Part model, mm, in its own coordinate system. A direction names the side the tool comes from. Give positions to 0.01 mm unless a question says otherwise; leave off trailing zeros. Write each loop counter-clockwise with the first axis right and the second up, starting at its lowest first coordinate (ties: lowest second). Pieces come first, ordered by that corner, then holes.
```python
from build123d import *

# Parameters (mm, degrees)
F0_R     = 1.778
F1_DEPTH = 2.159
F2_DEPTH = 6.35


with BuildPart() as f1:
    # F0 (on Front) → F1 (new body)
    with BuildSketch(Plane.XZ):
        Polygon((-13.906726, -6.464459), (-13.906726, -13.791269), (7.429274, -13.791269), (7.429274, -6.464459), (-1.206726, -6.464459), align=None)
        with Locations((-9.588726, -10.127864)):
            Circle(F0_R, mode=Mode.SUBTRACT)
        with Locations((3.111274, -10.127864)):
            Circle(F0_R, mode=Mode.SUBTRACT)
        Polygon((-16.446726, -13.791269), (-13.906726, -13.791269), (-13.906726, -6.464459), (-16.126592, -6.464459), (-16.446726, -7.197061), align=None)
        Polygon((-16.126592, -6.464459), (-13.906726, -6.464459), (-2.316659, 20.058554), (-1.206726, 20.058554), (-1.206726, -6.464459), (7.429274, -6.464459), (7.429274, 22.598554), (-1.206726, 22.598554), (-3.426592, 22.598554), (-13.906726, -1.384459), align=None)
        Polygon((-2.316659, 20.058554), (-13.906726, -6.464459), (-1.206726, -6.464459), (-1.206726, 20.058554), align=None)
    extrude(amount=F1_DEPTH)

    # F0 (on Front) → F2 (join)
    with BuildSketch(Plane.XZ):
        Polygon((-16.126592, -6.464459), (-13.906726, -6.464459), (-2.316659, 20.058554), (-1.206726, 20.058554), (-1.206726, -6.464459), (7.429274, -6.464459), (7.429274, 22.598554), (-1.206726, 22.598554), (-3.426592, 22.598554), (-13.906726, -1.384459), align=None)
        Polygon((-16.446726, -13.791269), (-13.906726, -13.791269), (-13.906726, -6.464459), (-16.126592, -6.464459), (-16.446726, -7.197061), align=None)
    extrude(amount=F2_DEPTH)


solid = f1.part
```
1) Wall check: L1, parallel to X at y = -1.25, z = -11.5; L2, parallel to Z at x = -10, y = -1.5; L3, parallel to X at y = -3, z = 2. Give the ranges that are in metal, low to high.
Answers follow:
L1: x = -16.45 to -10.72, -8.46 to 1.98, 4.24 to 7.43
L2: z = -13.79 to -11.86, -8.4 to 7.56
L3: x = -12.43 to -10.21, -1.21 to 7.43
2) Saw through at B-B, the plane x = -9.25. Write the cut outline in (y, z), then the cut area to 3 significant figures.
Answers follow:
outline: (-6.35, 4.19) - (-2.16, 4.19) - (-2.16, -8.38) - (0, -8.38) - (0, 9.27) - (-6.35, 9.27) - close; (-2.16, -13.79) - (0, -13.79) - (0, -11.87) - (-2.16, -11.87) - close
area: 63.5 mm2
3) 3-axis set-ups, long thin cutter, end or side, ignore diameter. For faces 4 (the face through (1, -6.35, 9)), 5 (the face through (-13.907, -4, -10)), 6 (the face through (-2, -4, 20.059)): which of +Z, -Z, +X, -X, +Y, -Y reach the whole face in a straight line?
Answers follow:
face 4: +Z, -Z, +X, -X, -Y
face 5: -Z, +X, -Y
face 6: -Z, -Y
4) Saw through at D-D, the plane z = -3. Write the cut outline in (x, y).
Answers follow:
outline: (-14.61, -6.35) - (-12.39, -6.35) - (-12.39, -2.16) - (-1.21, -2.16) - (-1.21, -6.35) - (7.43, -6.35) - (7.43, 0) - (-14.61, 0) - close
5) Two-plate mould, pull along Z, no slides. Class faces 1 (the face through (2, -3, 22.599)), 2 (the face through (3, -4, -6.464)), 3 (the face through (2.726, -1.064, -11.864)): +Z half, -Z half, draft (parallel to the pull), parting line (faces both ways), or undercut.
Answers follow:
face 1: +Z half
face 2: -Z half
face 3: undercut
6) Pin check, flat tips, straight feed: pin 1 Ø4 at (x, z) = (3.11, -10.13) entering from -Y; pin 2 Ø3 at (y, z) = (-5.5, -4) entering from -X; pin 3 Ø1.5 at (y, z) = (-5, -3) entering from -X; pin 4 Ø4 at (x, z) = (-9.59, -10.13) entering from +Y. Stop position of each tip, or through.
Answers follow:
pin 1: stops at y = -2.16
pin 2: stops at x = -15.71
pin 3: stops at x = -14.94
pin 4: stops at y = 0
7) Saw through at A-A, the plane y = -1.5. Write the cut outline in (x, z).
Answers follow:
outline: (-16.45, -13.79) - (7.43, -13.79) - (7.43, 22.6) - (-3.43, 22.6) - (-16.13, -6.46) - (-16.45, -7.2) - close; hole circle Ø3.56 at (-9.59, -10.13); hole circle Ø3.56 at (3.11, -10.13)
8) Saw through at C-C, the plane y = -3.25. Write the cut outline in (x, z), then the cut area to 3 significant figures.
Answers follow:
outline: (-16.45, -13.79) - (-13.91, -13.79) - (-13.91, -6.46) - (-2.32, 20.06) - (-1.21, 20.06) - (-1.21, -6.46) - (7.43, -6.46) - (7.43, 22.6) - (-3.43, 22.6) - (-16.13, -6.46) - (-16.45, -7.2) - close
area: 335 mm2
